Answer from the drawing. Dimensions are ordinates in mm from the lowest x, y and z of the part. Give positions to 0.01 mm unless a question says otherwise; leave off trailing zeros. Loops run counter-clockwise (first coordinate to the right, second up) from the corner with the lowest first, then second, coordinate; pieces in that order, holes last. Notation, with made-up numbers: (-7.5, 21) -> (22.5, 21) arc R14 cw to (22.5, 39) -> close; hole circle Ø2 at (15.25, 66). An arc over 180 degrees is marked (long way). Return JSON: item names as keys, results as strings. Group by question number.
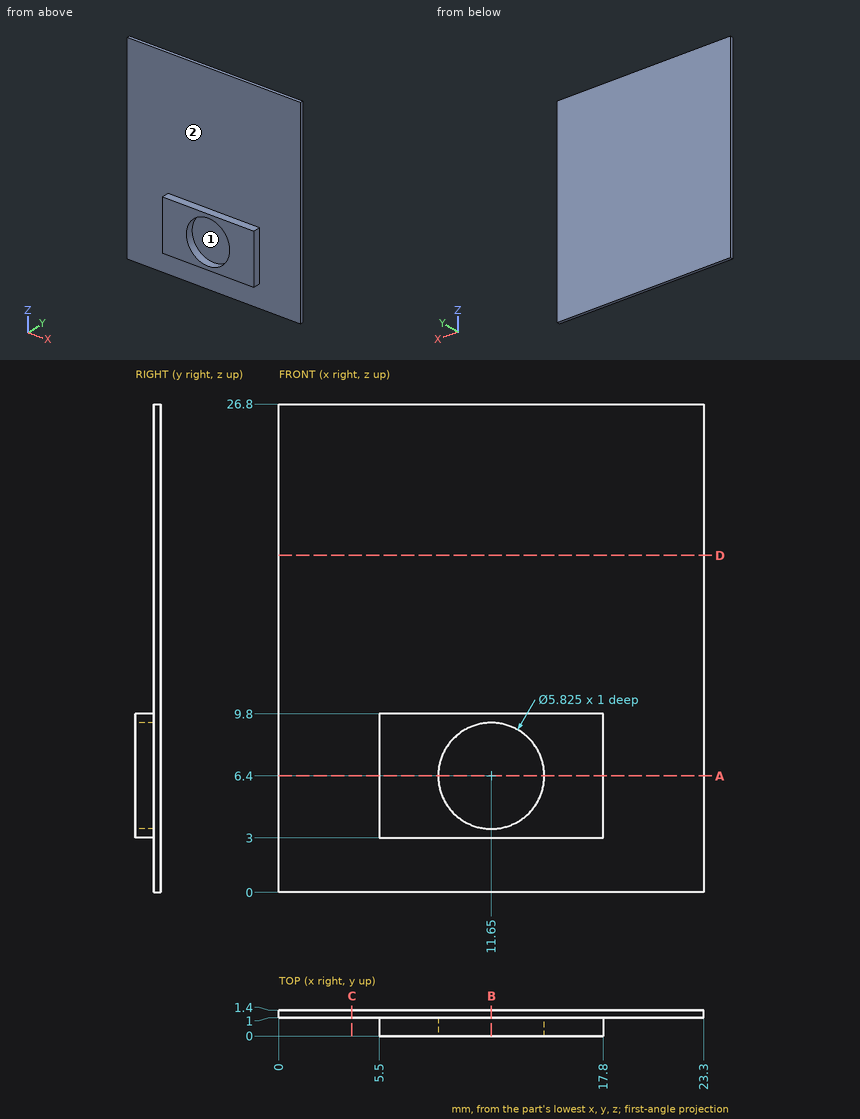
1. Section A-A on z = 6.4 is taken. Determine the outline of the cut face in (x, y), then the cut area to 3 significant figures.
2. Section D-D on z = 18.5 is taken. Determine the outline of the cut face in (x, y).
3. Flat-ended cylindrical pins translate along their axes: pin 1 Ø0.5 at (x, y) = (12.5, 0.5) entering from -Z; pin 2 Ø1.7 at (x, z) = (10.5, 5) entering from -Y; pin 3 Ø0.5 at (x, y) = (12.5, 0.5) entering from +Z. Find the tip coordinate at first contact, or state that the pin passes through.
4. Section B-B on x = 11.65 is taken. Determine the outline of the cut face in (y, z), then the cut area to 3 significant figures.
5. Straight lines are drawn through the part: line 1 (Z direction, x = 11.65, y = 0.4); line 2 (Y direction, x = 2.75, z = 24.5); line 3 (X direction, y = 0.9, z = 4.75). For each, find the intervals that lie inside material, in ascending order. Write a range as from..to.
6. Section C-C on x = 4 is taken. Determine the outline of the cut face in (y, z).
7. Determine the mould class of the marked faces 1 and 2 for opening direction Z: pulls with the +Z half, pulls with the -Z half, needs draft (parallel to the pull), parting line crosses it, or undercut.
Completed:
{
 "1": {"outline": "(0, 1) -> (5.5, 1) -> (5.5, 0) -> (8.74, 0) -> (8.74, 1) -> (14.56, 1) -> (14.56, 0) -> (17.8, 0) -> (17.8, 1) -> (23.3, 1) -> (23.3, 1.4) -> (0, 1.4) -> close", "area": "15.8 mm²"},
 "2": {"outline": "(0, 1) -> (23.3, 1) -> (23.3, 1.4) -> (0, 1.4) -> close"},
 "3": {"pin 1": "stops at z = 3", "pin 2": "stops at y = 1", "pin 3": "stops at z = 9.8"},
 "4": {"outline": "(0, 3) -> (1, 3) -> (1, 0) -> (1.4, 0) -> (1.4, 26.8) -> (1, 26.8) -> (1, 9.8) -> (0, 9.8) -> (0, 9.31) -> (1, 9.31) -> (1, 3.49) -> (0, 3.49) -> close", "area": "11.7 mm²"},
 "5": {"line 1": "z = 3..3.49, 9.31..9.8", "line 2": "y = 1..1.4", "line 3": "x = 5.5..9.25, 14.05..17.8"},
 "6": {"outline": "(1, 0) -> (1.4, 0) -> (1.4, 26.8) -> (1, 26.8) -> close"},
 "7": {"face 1": "undercut", "face 2": "needs draft"}
}
